from build123d import *

# Parameters (mm, degrees)
SKETCH1_W            = 110
SKETCH1_H            = 60
BOSS_EXTRUDE1_DEPTH  = 10
SKETCH2_W            = 93.6
SKETCH2_H            = 43.6
BOSS_EXTRUDE3_DEPTH  = 7
SKETCH3_W            = 21.7
SKETCH3_H            = 23.4
CUT_EXTRUDE1_DEPTH   = 7
FILLET1_R            = 12
FILLET1_OF_MIRROR1_R = 12


with BuildPart() as part:
    # Sketch1 → Boss-Extrude1 (new body)
    with BuildSketch(Plane.XY):
        with Locations((55, 30)):
            Rectangle(SKETCH1_W, SKETCH1_H)
    extrude(amount=BOSS_EXTRUDE1_DEPTH)

    # Sketch2 → Boss-Extrude3 (add)
    with BuildSketch(Plane.XY.offset(10)):
        with Locations((55, 30)):
            Rectangle(SKETCH2_W, SKETCH2_H)
    extrude(amount=BOSS_EXTRUDE3_DEPTH)

    # Sketch3 → Cut-Extrude1 (cut)
    with BuildSketch(Plane.XY.offset(17)):
        with Locations((37.25, 19.9)):
            Rectangle(SKETCH3_W, SKETCH3_H)
    cut_extrude1 = extrude(amount=-CUT_EXTRUDE1_DEPTH, mode=Mode.SUBTRACT)

    # Fillet1
    fillet1_edges = [part.edges().sort_by_distance(p)[0] for p in [
        (26.4, 31.6, 13.5),
    ]]
    fillet(fillet1_edges, radius=FILLET1_R)

    # Mirror1: Cut-Extrude1 across plane
    add(cut_extrude1.mirror(Plane(origin=(55, 0, 0), x_dir=(0, 0, 1), z_dir=(1, 0, 0))), mode=Mode.SUBTRACT)

    # Fillet1 of Mirror1
    fillet1_of_mirror1_edges = [part.edges().sort_by_distance(p)[0] for p in [
        (83.6, 31.6, 13.5),
    ]]
    fillet(fillet1_of_mirror1_edges, radius=FILLET1_OF_MIRROR1_R)


solid = part.part
Verification items for the finished model (mm, model axes). A direction names the side the tool comes from. Give positions to 0.01 mm unless a question says otherwise; leave off trailing zeros. Write each loop counter-clockwise with the first axis right and the second up, starting at its lowest first coordinate (ties: lowest second). Pieces come first, ordered by that corner, then holes.
(1) Access from +Z, -Z, +X, -X, +Y, -Y to the whole of each face (thin tool, end or side, straight path). Record for faces 1 (the face through (8.2, 30, 13)), 2 (the face through (43, 31.6, 14)), 3 (the face through (93, 8.2, 13)).
(2) Material ranges on line 1 (X direction, y = 17, z = 12.75); line 2 (X direction, y = 46, z = 12); line 3 (Z direction, x = 67, y = 5), recorded low to high.
(3) Cross-section at B-B (z = 12). Enter the section's corners in (x, y).
(4) Cross-section at D-D (y = 18). Enter the section's corners in (x, z).
(5) Mould release check, pull along X, two halves, no side actions. Record for faces 4 (the face through (101.8, 30, 13)), 5 (the face through (17, 8.2, 13)), 6 (the face through (48.1, 20, 14)): +X half, -X half, draft (parallel to the pull), parting line (faces both ways), or undercut.
(6) Cross-section at C-C (y = 44). Enter the section's corners in (x, z), plus the area to 3 significant figures.
(7) Gauge pin test, flat ends, axial feed: pin 1 (10 mm diameter, centred on y = 18.5, z = 12, fed in from +X); pin 2 (2 mm diameter, centred on x = 67, z = 15, fed in from -Y); pin 3 (2 mm diameter, centred on x = 15.5, z = 12, fed in from -Y); pin 4 (3.5 mm diameter, centred on y = 21, z = 12, fed in from +X). Record the tip position at first contact, or that the pin passes through.
(8) Cross-section at A-A (x = 88). Enter the section's corners in (y, z), plus the area to 3 significant figures.
Worked out:
1. face 1: +Z, -X, +Y, -Y
1. face 2: +Z, -Y
1. face 3: +Z, +X, -X, -Y
2. line 1: x = 8.2 to 26.4, 48.1 to 61.9, 83.6 to 101.8
2. line 2: x = 8.2 to 101.8
2. line 3: z = 0 to 10
3. outline: (8.2, 8.2) - (26.4, 8.2) - (26.4, 19.6) arc R12 cw to (38.4, 31.6) - (48.1, 31.6) - (48.1, 8.2) - (61.9, 8.2) - (61.9, 31.6) - (71.6, 31.6) arc R12 cw to (83.6, 19.6) - (83.6, 8.2) - (101.8, 8.2) - (101.8, 51.8) - (8.2, 51.8) - close
4. outline: (0, 0) - (110, 0) - (110, 10) - (101.8, 10) - (101.8, 17) - (83.6, 17) - (83.6, 10) - (61.9, 10) - (61.9, 17) - (48.1, 17) - (48.1, 10) - (26.4, 10) - (26.4, 17) - (8.2, 17) - (8.2, 10) - (0, 10) - close
5. face 4: +X half
5. face 5: draft
5. face 6: undercut
6. outline: (0, 0) - (110, 0) - (110, 10) - (101.8, 10) - (101.8, 17) - (8.2, 17) - (8.2, 10) - (0, 10) - close
6. area: 1,760 mm2
7. pin 1: stops at x = 110
7. pin 2: stops at y = 31.6
7. pin 3: stops at y = 8.2
7. pin 4: stops at x = 101.8
8. outline: (0, 0) - (60, 0) - (60, 10) - (51.8, 10) - (51.8, 17) - (8.2, 17) - (8.2, 10) - (0, 10) - close
8. area: 905 mm2
